Could you check a few things on this model? Use its own coordinates, in mm. Face numbers are marked on the shaded views. Round coordinates to 2 decimals unless told otherwise and drop trailing zeros. Use one line per item in the form item = value.
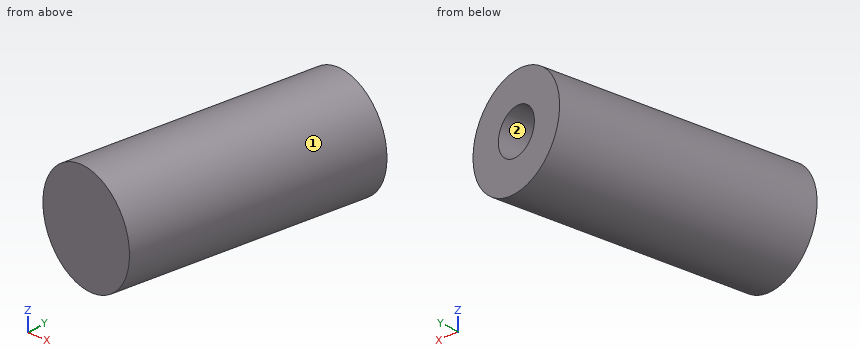
```python
from build123d import *

# Parameters (mm, degrees)
CYLINDER038_R               = 1.25
CYLINDER038_DEPTH           = 14
CYLINDER038_ROLL_ANGLE      = -89.999776
CYLINDER038_PITCH_ANGLE     = 1.4e-05
CYLINDER038_PLACEMENT_ANGLE = -9.999925
CYLINDER027_R               = 3
CYLINDER027_DEPTH           = 14
CYLINDER027_ROLL_ANGLE      = -89.999776
CYLINDER027_PITCH_ANGLE     = 1.4e-05
CYLINDER027_PLACEMENT_ANGLE = -9.999925


with BuildPart() as cylinder038:
    # Cylinder038 → Cylinder038 (new body)
    with BuildSketch(Plane.XY):
        Circle(CYLINDER038_R)
    extrude(amount=CYLINDER038_DEPTH)


with BuildPart() as cylinder038_1:
    # Cylinder038 roll: moved
    add(cylinder038.part.rotate(Axis((0, 0, 0), (1, 0, 0)), CYLINDER038_ROLL_ANGLE))


with BuildPart() as cylinder038_2:
    # Cylinder038 pitch: moved
    add(cylinder038_1.part.rotate(Axis((0, 0, 0), (0, 1, 0)), CYLINDER038_PITCH_ANGLE))


with BuildPart() as cylinder038_3:
    # Cylinder038 placement: moved
    add(cylinder038_2.part.moved(Location((32.055183, -23.766017, 7.500006))).rotate(Axis((32.055183, -23.766017, 7.500006), (0, 0, 1)), CYLINDER038_PLACEMENT_ANGLE))


with BuildPart() as cut032:
    # Cylinder027 → Cylinder027 (new body)
    with BuildSketch(Plane.XY):
        Circle(CYLINDER027_R)
    extrude(amount=CYLINDER027_DEPTH)


with BuildPart() as cut032_1:
    # Cylinder027 roll: moved
    add(cut032.part.rotate(Axis((0, 0, 0), (1, 0, 0)), CYLINDER027_ROLL_ANGLE))


with BuildPart() as cut032_2:
    # Cylinder027 pitch: moved
    add(cut032_1.part.rotate(Axis((0, 0, 0), (0, 1, 0)), CYLINDER027_PITCH_ANGLE))


with BuildPart() as cut032_3:
    # Cylinder027 placement: moved
    add(cut032_2.part.moved(Location((31.710772, -25.735381, 7.500001))).rotate(Axis((31.710772, -25.735381, 7.500001), (0, 0, 1)), CYLINDER027_PLACEMENT_ANGLE))

    # Cut032: cut Cylinder038
    add(cylinder038_3.part, mode=Mode.SUBTRACT)


solid = cut032_3.part
```
1. We'd pull the mould along X, two halves only. Please class the marked faces 1 and 2: +X half, -X half, draft (parallel to the pull), parting line (faces both ways), or undercut.
Solution:
face_1 = parting line
face_2 = undercut
2. Please list where these lines run through material, in increasing order: line 1 along X through (y, z) = (-12.5, 7); line 2 along X through (y, z) = (-17.5, 8.5); line 3 along Z through (x, y) = (35.75, -17.5).
Solution:
line_1 = 31.04 to 32.88, 35.2 to 37.05
line_2 = 30.29 to 32.4, 33.92 to 36.03
line_3 = 5.92 to 9.08
3. For P1, Ø2, axis at x = 36, y = -15.5, coming from the -Z side; P2, Ø3, axis at y = -17.5, z = 9, coming from the -X side; P3, Ø1, axis at x = 31.5, y = -20.5, coming from the +Z side, each with a flat end and sliding along its axis, tell me the tip position at first contact or that it passes through.
Solution:
P1 = 4.87
P2 = 29.96
P3 = 10.44
